from build123d import *

# Parameters (mm, degrees)
CUT_EXTRUDE1_START     = -6.244997998
CUT_EXTRUDE1_OUTLINE_W = 16
CUT_EXTRUDE1_OUTLINE_H = 4
CUT_EXTRUDE1_DEPTH     = 12.489995996
CUT_EXTRUDE2_REACH     = 17.1
SKETCH3_R              = 4


# Read off the part's stored shape, not the designer's step: Cut-Extrude1
with BuildPart() as part:
    # Sketch1 → Revolve1 (revolve)
    with BuildSketch(Plane.XY):
        with BuildLine():
            Line((0, 8), (0, -8))
            ThreePointArc((0, -8), (-8, 0), (0, 8))
        make_face()
    revolve(axis=Axis((0, 8, 0), (0, -1, 0)))

    # Cut-Extrude1 outline → Cut-Extrude1 (cut)
    with BuildSketch(Plane.XY.offset(CUT_EXTRUDE1_START)):
        with Locations((0, -7)):
            Rectangle(CUT_EXTRUDE1_OUTLINE_W, CUT_EXTRUDE1_OUTLINE_H)
        with Locations((0, 7)):
            Rectangle(CUT_EXTRUDE1_OUTLINE_W, CUT_EXTRUDE1_OUTLINE_H)
    extrude(amount=CUT_EXTRUDE1_DEPTH, mode=Mode.SUBTRACT)

    # Sketch3 → Cut-Extrude2 (cut, up to next)
    with BuildSketch(Plane(origin=(0, 5, 0), x_dir=(1, 0, 0), z_dir=(0, 1, 0)), mode=Mode.PRIVATE) as cut_extrude2_sk1:
        with Locations(Location((0, 0, 0), (0, 0, 270))):
            Circle(SKETCH3_R)
    cut_extrude2_tool1 = extrude(cut_extrude2_sk1.sketch, amount=-CUT_EXTRUDE2_REACH, mode=Mode.PRIVATE) & part.part
    add(cut_extrude2_tool1.solids().sort_by_distance((0, 5, 0))[0], mode=Mode.SUBTRACT)


solid = part.part
Read the model definition and answer for the solid it produces. Units are mm, in the model's axes. Coordinates: 2 decimals unless noted, no trailing zeros. Write each loop counter-clockwise with the first axis right and the second up, starting at its lowest first coordinate (ties: lowest second). Pieces come first, ordered by that corner, then holes. Notation, with made-up numbers: (-18.5, 14) -> (18.5, 14) arc R31 cw to (18.5, 53) -> close; hole circle Ø6 at (-3, 63.25). An arc over 180 degrees is marked (long way). Return JSON: item names as keys, results as strings.
(1) This flat-tipped pin is pushed along its axis until it touches: P1, Ø3, axis at x = -3.5, y = 3.5, coming from the -Z side. Where does it stop, or does it pass through?
Answers below:
{"P1": "z = -7.22"}
(2) The part is cut by section B-B on x = -1.25. Give the vertices of the cut face in (y, z), then the cut area to 3 significant figures.
Answers below:
{"outline": "(-5, -6.12) arc R7.9 ccw to (5, -6.12) -> (5, -3.8) -> (-5, -3.8) -> close; (-5, 3.8) -> (5, 3.8) -> (5, 6.12) arc R7.9 ccw to (-5, 6.12) -> close", "area": "70.7 mm^2"}
(3) The part is cut by section A-A on z = 0. Give the vertices of the cut face in (x, y) (3 decimals).
Answers below:
{"outline": "(-6.245, -5) -> (-4, -5) -> (-4, 5) -> (-6.245, 5) arc R8 ccw to start; (4, -5) -> (6.245, -5) arc R8 ccw to (6.245, 5) -> (4, 5) -> close"}
(4) Consider line 1 along X through (y, z) = (-0.25, -2.75); line 2 along X through (y, z) = (0.75, 0); line 3 along Z through (x, y) = (2, -4.25). Determine where each line is inside the solid, lowest interval first. Write a range as from..to.
Answers below:
{"line 1": "-7.51..-2.9, 2.9..7.51", "line 2": "-7.96..-4, 4..7.96", "line 3": "-6.48..-3.46, 3.46..6.48"}
(5) For a pull along X with two mould halves and no side action, classify faces 1 (the flat face through (1.3, -5, 4.1)), 2 (the cylindrical face through (-3.905, 0.07, -0.867)) as pulls with the +X half, pulls with the -X half, needs draft (parallel to the pull), parting line crosses it, or undercut.
Answers below:
{"face 1": "needs draft", "face 2": "undercut"}
(6) The part is cut by section D-D on z = 6.5. Give the vertices of the cut face in (x, y).
Answers below:
{"outline": "circle Ø9.33 at (0, 0)"}
(7) The part is cut by section C-C on y = -1. Give the vertices of the cut face in (x, z), then the cut area to 3 significant figures.
Answers below:
{"outline": "circle Ø15.87 at (0, 0); hole circle Ø8 at (0, 0)", "area": "148 mm^2"}
